from build123d import *

# Parameters (mm, degrees)
F1_DEPTH = 465
F2_W     = 31
F2_H     = 25
F3_DEPTH = 15.5
F4_W     = 31
F4_H     = 25
F5_DEPTH = 15.5
F6_R     = 2
F7_DEPTH = 10.001
F8_R     = 3.5
F9_DEPTH = 4
F10_R    = 1
F11_R    = 1


# Not quite as in the source:
# - a pattern or mirror of a feature is missing from the dataset's text; its kind, count and spacing are read off the source's solid


with BuildPart() as f1:
    # F0 (on Right) → F1 (new body, symmetric)
    with BuildSketch(Plane.YZ):
        Polygon((18.5, 12.5), (-18.5, 12.5), (-18.5, 2.5), (-15.5, 2.5), (-15.5, -22.5), (-10.5, -22.5), (-10.5, 2.5), (0, 2.5), (10.5, 2.5), (10.5, -22.5), (15.5, -22.5), (15.5, 2.5), (18.5, 2.5), align=None)
    extrude(amount=F1_DEPTH, both=True)

    # F2 (on face) → F3 (cut)
    with BuildSketch(Plane(origin=(-465, 0, 0), x_dir=(0, -1, 0), z_dir=(-1, 0, 0))):
        with Locations((0, -10)):
            Rectangle(F2_W, F2_H)
    extrude(amount=-F3_DEPTH, mode=Mode.SUBTRACT)

    # F4 (on face) → F5 (cut)
    with BuildSketch(Plane.YZ.offset(465)):
        with Locations((0, -10)):
            Rectangle(F4_W, F4_H)
    extrude(amount=-F5_DEPTH, mode=Mode.SUBTRACT)

    # F6 (on face) → F7 (cut, through all)
    with BuildSketch(Plane(origin=(0, 0, 2.5), x_dir=(1, 0, 0), z_dir=(0, 0, -1))):
        with Locations((-457.25, 9)):
            Circle(F6_R)
        with Locations((-457.25, -9)):
            Circle(F6_R)
    f7 = extrude(amount=-F7_DEPTH, mode=Mode.SUBTRACT)

    # F7_copies: F7 across plane
    add(f7.mirror(Plane(origin=(0, 0, 0), x_dir=(0, 0, 1), z_dir=(1, 0, 0))), mode=Mode.SUBTRACT)

    # F8 (on face) → F9 (cut)
    with BuildSketch(Plane.XY.offset(12.5)):
        with Locations((-457.25, -9)):
            Circle(F8_R)
        with Locations((-457.25, 9)):
            Circle(F8_R)
    f9 = extrude(amount=-F9_DEPTH, mode=Mode.SUBTRACT)

    # F9_copies: F9 across plane
    add(f9.mirror(Plane(origin=(0, 0, 0), x_dir=(0, 0, 1), z_dir=(1, 0, 0))), mode=Mode.SUBTRACT)

    # F10
    f10_edges = [f1.edges().sort_by_distance(p)[0] for p in [
        (465, 18.5, 7.5),
        (465, -18.5, 7.5),
        (449.5, 13, -22.5),
        (449.5, -13, -22.5),
        (-465, -18.5, 7.5),
        (-449.5, -13, -22.5),
        (-449.5, 13, -22.5),
        (-465, 18.5, 7.5),
    ]]
    fillet(f10_edges, radius=F10_R)

    # F11
    f11_edges = [f1.edges().sort_by_distance(p)[0] for p in [
        (-449.5, -10.5, -9.5),
        (-449.5, -15.5, -9.5),
        (-449.5, 15.5, -9.5),
        (-449.5, 10.5, -9.5),
        (-449.5, 13, -21.5),
        (-449.5, 13, 2.5),
        (-465, 0, 2.5),
        (-465, 0, 12.5),
        (0, -15.5, 2.5),
        (-464.707107, 18.207107, 12.5),
        (-464.707107, -18.207107, 12.5),
        (0, 18.5, 12.5),
        (0, -18.5, 12.5),
        (464.707107, 18.207107, 12.5),
        (464.707107, -18.207107, 12.5),
        (465, 0, 12.5),
        (-464.707107, 18.207107, 2.5),
        (-464.707107, -18.207107, 2.5),
        (0, 18.5, 2.5),
        (0, -18.5, 2.5),
        (464.707107, 18.207107, 2.5),
        (464.707107, -18.207107, 2.5),
        (465, 0, 2.5),
        (-449.5, -13, 2.5),
        (449.5, -13, 2.5),
        (0, -10.5, 2.5),
        (0, 10.5, 2.5),
        (449.5, 13, 2.5),
        (0, 15.5, 2.5),
        (449.5, -15.5, -9.5),
        (449.207107, -15.5, -22.207107),
        (0, -15.5, -22.5),
        (-449.207107, -15.5, -22.207107),
        (449.5, -10.5, -9.5),
        (0, -10.5, -22.5),
        (-449.207107, -10.5, -22.207107),
        (449.207107, -10.5, -22.207107),
        (449.5, 10.5, -9.5),
        (449.207107, 10.5, -22.207107),
        (0, 10.5, -22.5),
        (-449.207107, 10.5, -22.207107),
        (449.5, 15.5, -9.5),
        (0, 15.5, -22.5),
        (-449.207107, 15.5, -22.207107),
        (449.207107, 15.5, -22.207107),
    ]]
    fillet(f11_edges, radius=F11_R)


solid = f1.part
Geometry: final body of the model. Coordinates: model frame, mm. A direction names the side the tool comes from. Give positions to 0.01 mm unless a question says otherwise; leave off trailing zeros. Loops run counter-clockwise (first coordinate to the right, second up) from the corner with the lowest first, then second, coordinate; pieces in that order, holes last. Notation, with made-up numbers: M -2.75,32 L 7.25,32 A26 ccw 7.25,47 Z; hole C 44,-32.5 d5. An arc over 180 degrees is marked long. Put each result on its own line as item: value. Start each with the question number.
1) Contact query for flat-ended pins moving along their axis: pin 1 (1.5 mm diameter, centred on y = -13, z = -10, fed in from +X); pin 2 (4 mm diameter, centred on y = -9.5, z = -5, fed in from -X); pin 3 (3 mm diameter, centred on x = 457.25, y = -9, fed in from -Z); pin 4 (12 mm diameter, centred on x = -282, z = -6, fed in from -Y). Output: stop coordinate, or through.
2) Ray query, line 1 along Y through (x, z) = (457.25, 9.8); line 2 along Y through (x, z) = (-457.25, 3.95); line 3 along X through (y, z) = (-9, 6). Return the intervals inside material, ascending.
3) Cut plane B-B (x = 166.5). Output: boundary loops of the cut face in (y, z), then the cut area to 3 significant figures.
4) Cut plane A-A (z = -15). Output: boundary loops of the cut face in (x, y).
5) Access query for faces 4 (the flat face through (6, 10.5, -10)), 5 (the flat face through (6, -15.5, -10)). Directions: +Z, -Z, +X, -X, +Y, -Y. A direction counts if a zero-diameter tool reaches every point of the face in a straight line with its end or side. Return the directions, or none.
6) Pull-direction query (Y, two-part tool) for faces 1 (the flat face through (6, 0, 12.5)), 2 (the flat face through (6, 15.5, -10)), 3 (the flat face through (6, 0, 2.5)); classes: pulls with the +Y half, pulls with the -Y half, needs draft (parallel to the pull), parting line crosses it, or undercut.
Verdict:
1. pin 1: x = 449.5
1. pin 2: x = -449.5
1. pin 3: through
1. pin 4: y = -15.5
2. line 1: -18.5 to -12.5, -5.5 to 5.5, 12.5 to 18.5
2. line 2: -18.5 to -11, -7 to 7, 11 to 18.5
2. line 3: -465 to -459.25, -455.25 to 455.25, 459.25 to 465
3. outline: M -18.5,3.5 A1 ccw -17.5,2.5 L -16.5,2.5 A1 cw -15.5,1.5 L -15.5,-21.5 A1 ccw -14.5,-22.5 L -11.5,-22.5 A1 ccw -10.5,-21.5 L -10.5,1.5 A1 cw -9.5,2.5 L 9.5,2.5 A1 cw 10.5,1.5 L 10.5,-21.5 A1 ccw 11.5,-22.5 L 14.5,-22.5 A1 ccw 15.5,-21.5 L 15.5,1.5 A1 cw 16.5,2.5 L 17.5,2.5 A1 ccw 18.5,3.5 L 18.5,11.5 A1 ccw 17.5,12.5 L -17.5,12.5 A1 ccw -18.5,11.5 Z
3. area: 619 mm2
4. outline: M -449.5,-14.5 A1 ccw -448.5,-15.5 L 448.5,-15.5 A1 ccw 449.5,-14.5 L 449.5,-11.5 A1 ccw 448.5,-10.5 L -448.5,-10.5 A1 ccw -449.5,-11.5 Z; M -449.5,11.5 A1 ccw -448.5,10.5 L 448.5,10.5 A1 ccw 449.5,11.5 L 449.5,14.5 A1 ccw 448.5,15.5 L -448.5,15.5 A1 ccw -449.5,14.5 Z
5. face 4: -Z, +X, -X
5. face 5: -Z, +X, -X, -Y
6. face 1: needs draft
6. face 2: pulls with the +Y half
6. face 3: undercut
